Geometry check sheet. Reference: the model listing, model coordinates, mm. Round coordinates to 2 decimals unless told otherwise and drop trailing zeros. Write each loop counter-clockwise with the first axis right and the second up, starting at its lowest first coordinate (ties: lowest second). Pieces come first, ordered by that corner, then holes. Notation, with made-up numbers: M 77.5,38.5 L 128.5,38.5 A14 ccw 128.5,59.5 Z; hole C 34,-8 d1. An arc over 180 degrees is marked long. Use a Markdown table: item, result.
```python
from build123d import *

# Parameters (mm, degrees)
SKETCH1_R           = 7.75
SKETCH1_R_2         = 1.75
BOSS_EXTRUDE1_DEPTH = 3.175


with BuildPart() as part:
    # Sketch1 → Boss-Extrude1 (new body)
    with BuildSketch(Plane(origin=(0, 0, 0), x_dir=(1, 0, 0), z_dir=(0, 1, 0))):
        with BuildLine():
            Line((-17.104001725, 6.625), (-2.814582562, -18.125))
            ThreePointArc((-2.814582562, -18.125), (0, -19.75), (2.814582562, -18.125))
            Line((2.814582562, -18.125), (17.104001725, 6.625))
            ThreePointArc((17.104001725, 6.625), (17.104001725, 9.875), (14.289419162, 11.5))
            Line((14.289419162, 11.5), (-14.289419162, 11.5))
            ThreePointArc((-14.289419162, 11.5), (-17.104001725, 9.875), (-17.104001725, 6.625))
        make_face()
        with Locations(Location((0, 0, 0), (0, 0, 270))):  # turned: the seam where the file's is
            Circle(SKETCH1_R, mode=Mode.SUBTRACT)
        with Locations(Location((-14.289419162, 8.25, 0), (0, 0, 270))):  # turned: the seam where the file's is
            Circle(SKETCH1_R_2, mode=Mode.SUBTRACT)
        with Locations(Location((0, -16.5, 0), (0, 0, 270))):  # turned: the seam where the file's is
            Circle(SKETCH1_R_2, mode=Mode.SUBTRACT)
        with Locations(Location((14.289419162, 8.25, 0), (0, 0, 270))):  # turned: the seam where the file's is
            Circle(SKETCH1_R_2, mode=Mode.SUBTRACT)
    extrude(amount=BOSS_EXTRUDE1_DEPTH)


solid = part.part
```
Item 1: Cross-section at B-B, the plane x = 0. Record the cut outline in (y, z) (3 decimals).
Outcome:
| item | result |
|---|---|
| outline | M 0,-11.5 L 3.175,-11.5 L 3.175,-7.75 L 0,-7.75 Z; M 0,7.75 L 3.175,7.75 L 3.175,14.75 L 0,14.75 Z; M 0,18.25 L 3.175,18.25 L 3.175,19.75 L 0,19.75 Z |
Item 2: Material ranges on line 1 along X through (y, z) = (1.85, -8.25); line 2 along Z through (x, y) = (-1.5, 0.95); line 3 along Z through (x, y) = (-4.5, 0.7), recorded low to high. Write a range as from..to.
Outcome:
| item | result |
|---|---|
| line 1 | x = -17.54..-16.04, -12.54..12.54, 16.04..17.54 |
| line 2 | z = -11.5..-7.6, 7.6..15.6, 17.4..19.38 |
| line 3 | z = -11.5..-6.31, 6.31..15.21 |
Item 3: Cross-section at A-A, the plane z = -8.25. Record the cut outline in (x, y) (3 decimals).
Outcome:
| item | result |
|---|---|
| outline | M -17.539,0 L -16.039,0 L -16.039,3.175 L -17.539,3.175 Z; M -12.539,0 L 12.539,0 L 12.539,3.175 L -12.539,3.175 Z; M 16.039,0 L 17.539,0 L 17.539,3.175 L 16.039,3.175 Z |
Item 4: Cross-section at D-D, the plane z = 0. Record the cut outline in (x, y) (3 decimals).
Outcome:
| item | result |
|---|---|
| outline | M -13.279,0 L -7.75,0 L -7.75,3.175 L -13.279,3.175 Z; M 7.75,0 L 13.279,0 L 13.279,3.175 L 7.75,3.175 Z |
Item 5: Cross-section at C-C, the plane y = 2.1. Record the cut outline in (x, z) (3 decimals).
Outcome:
| item | result |
|---|---|
| outline | M -17.104,-6.625 A3.25 ccw -14.289,-11.5 L 14.289,-11.5 A3.25 ccw 17.104,-6.625 L 2.815,18.125 A3.25 ccw -2.815,18.125 Z; hole C -14.289,-8.25 d3.5; hole C 0,0 d15.5; hole C 0,16.5 d3.5; hole C 14.289,-8.25 d3.5 |
Item 6: Mould release check, pull along X, two halves, no side actions. Record for faces 1 (the face through (0.526, 1.565, 18.169)), 2 (the face through (7.684, 1.565, -1.009)), 3 (the face through (9.86, 1.57, 5.92)), 4 (the face through (-8, 0, 0)): +X half, -X half, draft (parallel to the pull), parting line (faces both ways), or undercut.
Outcome:
| item | result |
|---|---|
| face 1 | undercut |
| face 2 | undercut |
| face 3 | +X half |
| face 4 | draft |
